from build123d import *

# Parameters (mm, degrees)
SKETCH_1_W          = 60
SKETCH_1_H          = 40
EXTRUDE_1_DEPTH     = 30
SKETCH_2_W          = 60
SKETCH_2_H          = 3.5
CUT_EXTRUDE_1_DEPTH = 24
SKETCH_3_W          = 2
SKETCH_3_H          = 40
CUT_EXTRUDE_2_DEPTH = 24
SKETCH_4_R          = 2.25
CUT_EXTRUDE_3_DEPTH = 47.904157598
SKETCH_5_R          = 4.25
CUT_EXTRUDE_4_DEPTH = 24


with BuildPart() as part:
    # 草图1 → 拉伸1 (new body)
    with BuildSketch(Plane(origin=(0, 0, 0), x_dir=(1, 0, 0), z_dir=(0, 1, 0))):
        Rectangle(SKETCH_1_W, SKETCH_1_H)
    extrude(amount=EXTRUDE_1_DEPTH)

    # 草图2 → 切除-拉伸1 (cut)
    with BuildSketch(Plane(origin=(0, 30, 0), x_dir=(-1, 0, 0), z_dir=(0, 1, 0))):
        with Locations((0, -16.75)):
            Rectangle(SKETCH_2_W, SKETCH_2_H)
        with Locations((0, -11.75)):
            Rectangle(SKETCH_2_W, SKETCH_2_H)
        with Locations((0, -6.75)):
            Rectangle(SKETCH_2_W, SKETCH_2_H)
        with Locations((0, -1.75)):
            Rectangle(SKETCH_2_W, SKETCH_2_H)
        with Locations((0, 3.25)):
            Rectangle(SKETCH_2_W, SKETCH_2_H)
        with Locations((0, 8.25)):
            Rectangle(SKETCH_2_W, SKETCH_2_H)
        with Locations((0, 13.25)):
            Rectangle(SKETCH_2_W, SKETCH_2_H)
        with Locations((0, 18.25)):
            Rectangle(SKETCH_2_W, SKETCH_2_H)
    extrude(amount=-CUT_EXTRUDE_1_DEPTH, mode=Mode.SUBTRACT)

    # 草图3 → 切除-拉伸2 (cut)
    with BuildSketch(Plane(origin=(0, 30, 0), x_dir=(-1, 0, 0), z_dir=(0, 1, 0))):
        with Locations((-17, 0)):
            Rectangle(SKETCH_3_W, SKETCH_3_H)
        with Locations((9.5, 0)):
            Rectangle(SKETCH_3_W, SKETCH_3_H)
    extrude(amount=-CUT_EXTRUDE_2_DEPTH, mode=Mode.SUBTRACT)

    # 草图4 → 切除-拉伸3 (cut, through all)
    with BuildSketch(Plane.XZ):
        with Locations(Location((14.15, 5, 0), (0, 0, 270))):
            Circle(SKETCH_4_R)
        with Locations(Location((-14.15, 5, 0), (0, 0, 180))):
            Circle(SKETCH_4_R)
    extrude(amount=-CUT_EXTRUDE_3_DEPTH, mode=Mode.SUBTRACT)

    # 草图5 → 切除-拉伸4 (cut)
    with BuildSketch(Plane(origin=(0, 30, 0), x_dir=(-1, 0, 0), z_dir=(0, 1, 0))):
        with Locations((14.15, 5)):
            Circle(SKETCH_5_R)
        with Locations((-14.15, 5)):
            Circle(SKETCH_5_R)
    extrude(amount=-CUT_EXTRUDE_4_DEPTH, mode=Mode.SUBTRACT)


solid = part.part
Source: CAD feature listing. Evaluate the final solid. Frame: model axes, mm. A direction names the side the tool comes from. Give positions to 0.01 mm unless a question says otherwise; leave off trailing zeros. Write each loop counter-clockwise with the first axis right and the second up, starting at its lowest first coordinate (ties: lowest second). Pieces come first, ordered by that corner, then holes. Notation, with made-up numbers: M -13.75,83 L 4.25,83 A27 cw 4.25,111 Z; hole C -22.5,30 d5. An arc over 180 degrees is marked long. Return JSON: item names as keys, results as strings. Group by question number.
1) Ray query, L1, parallel to X at y = 3.95, z = 5; L2, parallel to Z at x = -14.15, y = 4.6; L3, parallel to Y at x = -9.5, z = 6.5. Return the intervals inside material, ascending.
2) Cut plane B-B, the plane y = 14.75. Give the number of separate pieces and of enclosed holes in the cut face, then the cut area to 3 significant figures.
3) Draft query along Z for faces 1 (the face through (24, 18, 15)), 2 (the face through (-8.5, 18, 11)), 3 (the face through (24, 18, 16.5)), 4 (the face through (-14.11, 18.17, 0.75)). Return one class per face: released by +Z, released by -Z, zero draft, split by the parting line, or undercut.
4) First-contact query: pin 1 Ø15.5 at (x, y) = (-17, 19) entering from +Z. Flat tip, straight axial feed; report the tip coordinate or a pass-through.
5) Cut plane D-D, the plane z = 8.5. Output: boundary loops of the cut face in (x, y), then the cut area to 3 significant figures.
6) Set-up query: faces 5 (the face through (-20, 30, -19)), 6 (the face through (24, 18, 1.5)), 7 (the face through (-8.5, 18, -19)). Return all of +Z, -Z, +X, -X, +Y, -Y with unobstructed straight access to the full face (end or side cutting, diameter ignored); none if empty.
Data:
{
 "1": {"L1": "x = -30 to -16.4, -11.9 to 11.9, 16.4 to 30", "L2": "z = -20 to 2.75, 7.25 to 20", "L3": "y = 0 to 6"},
 "2": {"separate pieces": "24", "enclosed holes": "0", "area": "646 mm²"},
 "3": {"face 1": "undercut", "face 2": "zero draft", "face 3": "released by +Z", "face 4": "undercut"},
 "4": {"pin 1": "stops at z = 16.5"},
 "5": {"outline": "M -30,0 L 30,0 L 30,6 L -30,6 Z", "area": "360 mm²"},
 "6": {"face 5": "+Z, -Z, +X, -X, +Y", "face 6": "+X, -X, +Y", "face 7": "+Z, -Z, +Y"}
}
